from build123d import *

# Parameters (mm, degrees)
SKETCH1_R           = 50
BOSS_EXTRUDE1_DEPTH = 15
SKETCH2_R           = 5
CUT_EXTRUDE1_DEPTH  = 73.284161474
SKETCH3_R           = 25
SKETCH3_R_2         = 13
BOSS_EXTRUDE2_DEPTH = 60
SKETCH6_R           = 6
SKETCH6_R_2         = 17.5
BOSS_EXTRUDE3_DEPTH = 15
CUT_EXTRUDE2_START  = -30
SKETCH7_R           = 17.5
CUT_EXTRUDE2_DEPTH  = 30


with BuildPart() as part:
    # Sketch1 → Boss-Extrude1 (new body)
    with BuildSketch(Plane(origin=(0, 0, 0), x_dir=(1, 0, 0), z_dir=(0, 1, 0))):
        with Locations(Location((0, 0, 0), (0, 0, 270))):
            Circle(SKETCH1_R)
    extrude(amount=BOSS_EXTRUDE1_DEPTH)

    # Sketch2 → Cut-Extrude1 (cut, through all)
    with BuildSketch(Plane(origin=(0, 15, 0), x_dir=(1, 0, 0), z_dir=(0, 1, 0))):
        with Locations(Location((0, 35, 0), (0, 0, 270))):
            Circle(SKETCH2_R)
        with Locations(Location((30.310889132, 17.5, 0), (0, 0, 270))):
            Circle(SKETCH2_R)
        with Locations(Location((30.310889132, -17.5, 0), (0, 0, 270))):
            Circle(SKETCH2_R)
        with Locations(Location((0, -35, 0), (0, 0, 270))):
            Circle(SKETCH2_R)
        with Locations(Location((-30.310889132, -17.5, 0), (0, 0, 270))):
            Circle(SKETCH2_R)
        with Locations(Location((-30.310889132, 17.5, 0), (0, 0, 270))):
            Circle(SKETCH2_R)
    extrude(amount=-CUT_EXTRUDE1_DEPTH, mode=Mode.SUBTRACT)

    # Sketch3 → Boss-Extrude2 (add)
    with BuildSketch(Plane(origin=(0, 15, 0), x_dir=(1, 0, 0), z_dir=(0, 1, 0))):
        with Locations(Location((0, 0, 0), (0, 0, 270))):
            Circle(SKETCH3_R)
        with Locations(Location((0, 0, 0), (0, 0, 270))):
            Circle(SKETCH3_R_2, mode=Mode.SUBTRACT)
    extrude(amount=BOSS_EXTRUDE2_DEPTH)

    # Sketch6 → Boss-Extrude3 (add)
    with BuildSketch(Plane(origin=(0, 75, 0), x_dir=(1, 0, 0), z_dir=(0, 1, 0))):
        with BuildLine():
            Line((14.309088021, 54.5), (28.618176043, 9))
            ThreePointArc((28.618176043, 9), (30, 0), (28.618176043, -9))
            Line((28.618176043, -9), (14.309088021, -54.5))
            ThreePointArc((14.309088021, -54.5), (0, -65), (-14.309088021, -54.5))
            Line((-14.309088021, -54.5), (-28.618176043, -9))
            ThreePointArc((-28.618176043, -9), (-30, 0), (-28.618176043, 9))
            Line((-28.618176043, 9), (-14.309088021, 54.5))
            ThreePointArc((-14.309088021, 54.5), (0, 65), (14.309088021, 54.5))
        make_face()
        with Locations(Location((0, -50, 0), (0, 0, 270))):
            Circle(SKETCH6_R, mode=Mode.SUBTRACT)
        with Locations(Location((0, 50, 0), (0, 0, 270))):
            Circle(SKETCH6_R, mode=Mode.SUBTRACT)
        with Locations(Location((0, 0, 0), (0, 0, 270))):
            Circle(SKETCH6_R_2, mode=Mode.SUBTRACT)
    extrude(amount=BOSS_EXTRUDE3_DEPTH)

    # Sketch7 → Cut-Extrude2 (cut)
    with BuildSketch(Plane(origin=(0, 90, 0), x_dir=(1, 0, 0), z_dir=(0, 1, 0)).offset(CUT_EXTRUDE2_START)):
        with Locations(Location((0, 0, 0), (0, 0, 270))):
            Circle(SKETCH7_R)
    extrude(amount=CUT_EXTRUDE2_DEPTH, mode=Mode.SUBTRACT)


solid = part.part
Verification items for the finished model (mm, model axes). A direction names the side the tool comes from. Round coordinates to 2 decimals unless told otherwise and drop trailing zeros. Loops run counter-clockwise (first coordinate to the right, second up) from the corner with the lowest first, then second, coordinate; pieces in that order, holes last. Notation, with made-up numbers: (-33.5, 24.5) - (-18.5, 24.5) arc R11 ccw to (-18.5, 42.5) - close; hole circle Ø9 at (35.25, -35.75). An arc over 180 degrees is marked (long way). Use a Markdown table: item, result. Add a question column.
1. Release check for a two-part mould opening along X. For faces 1 (the face through (34.527, 7.605, 20.188)), 2 (the face through (-21.363, 82.395, 32.068)), 3 (the face through (0, 82, 65)), 4 (the face through (21.363, 82.395, -32.068)) record: released by +X, released by -X, zero draft, split by the parting line, or undercut.
2. Section check D-D, the plane z = 0. Record the boundary of the cut face in (x, y), plus the area to 3 significant figures.
3. Access from +Z, -Z, +X, -X, +Y, -Y to the whole of each face (thin tool, end or side, straight path). Record for faces 5 (the face through (22.9, 15, 10.4)), 6 (the face through (0, 82, -56)), 7 (the face through (-35.192, 7.605, 16.416)).
4. Section check A-A, the plane y = 12.5. Record the boundary of the cut face in (x, z), plus the area to 3 significant figures.
5. Section check B-B, the plane z = -14.5. Record the boundary of the cut face in (x, y).
6. Section check C-C, the plane x = 0. Give the number of separate pieces and of enclosed holes in the cut face, plus the area to 3 significant figures.
7. Gauge pin test, flat ends, axial feed: pin 1 (6 mm diameter, centred on y = 77, z = 10, fed in from -X); pin 2 (12 mm diameter, centred on x = 13, y = 76.5, fed in from +Z); pin 3 (8 mm diameter, centred on x = 0, z = -35, fed in from -Y). Record the tip position at first contact, or that the pin passes through.
8. Thickness scan on probe 1 along Y at (x, z) = (-6.5, -27); probe 2 along Z at (x, y) = (0.5, 81); probe 3 along X at (y, z) = (33, 0). Record the ranges inside material, lowest first. Write a range as [from, to].
Checks:
| question | item | result |
|---|---|---|
| 1 | face 1 | undercut |
| 1 | face 2 | released by -X |
| 1 | face 3 | split by the parting line |
| 1 | face 4 | released by +X |
| 2 | outline | (-50, 0) - (50, 0) - (50, 15) - (25, 15) - (25, 75) - (30, 75) - (30, 90) - (17.5, 90) - (17.5, 60) - (13, 60) - (13, 15) - (-13, 15) - (-13, 60) - (-17.5, 60) - (-17.5, 90) - (-30, 90) - (-30, 75) - (-25, 75) - (-25, 15) - (-50, 15) - close |
| 2 | area | 3,180 mm^2 |
| 3 | face 5 | none |
| 3 | face 6 | +Y |
| 3 | face 7 | -Y |
| 4 | outline | circle Ø100 at (0, 0); hole circle Ø10 at (-30.31, -17.5); hole circle Ø10 at (-30.31, 17.5); hole circle Ø10 at (0, -35); hole circle Ø10 at (0, 35); hole circle Ø10 at (30.31, -17.5); hole circle Ø10 at (30.31, 17.5) |
| 4 | area | 7,380 mm^2 |
| 5 | outline | (-47.85, 0) - (-34.31, 0) - (-34.31, 15) - (-47.85, 15) - close; (-26.89, 75) - (-20.37, 75) - (-20.37, 15) - (-26.31, 15) - (-26.31, 0) - (26.31, 0) - (26.31, 15) - (20.37, 15) - (20.37, 75) - (26.89, 75) - (26.89, 90) - (9.8, 90) - (9.8, 60) - (-9.8, 60) - (-9.8, 90) - (-26.89, 90) - close; (34.31, 0) - (47.85, 0) - (47.85, 15) - (34.31, 15) - close |
| 6 | separate pieces | 5 |
| 6 | enclosed holes | 0 |
| 6 | area | 3,570 mm^2 |
| 7 | pin 1 | stops at x = -29.17 |
| 7 | pin 2 | stops at z = 63.27 |
| 7 | pin 3 | stops at y = 75 |
| 8 | probe 1 | y = [0, 15], [75, 90] |
| 8 | probe 2 | z = [-64.99, -55.98], [-44.02, -17.49], [17.49, 44.02], [55.98, 64.99] |
| 8 | probe 3 | x = [-25, -13], [13, 25] |
